Autodesk Inventor part; units mm, degrees
ref_plane "YZ Plane" through (0, 0, 0) normal (1, 0, 0) x (0, 1, 0)
ref_plane "XZ Plane" through (0, 0, 0) normal (0, 1, 0) x (-1, 0, 0)
ref_plane "XY Plane" through (0, 0, 0) normal (0, 0, 1) x (1, 0, 0)
sketch "Skizze1" plane through (0, 0, 0) normal (0, 1, 0) x (-1, 0, 0)
  line L0 (0, 6.5) -> (5.6292, 3.25)
  line L1 (5.6292, 3.25) -> (5.6292, -3.25)
  line L2 (5.6292, -3.25) -> (0, -6.5)
  line L3 (0, -6.5) -> (-5.6292, -3.25)
  line L4 (-5.6292, -3.25) -> (-5.6292, 3.25)
  line L5 (-5.6292, 3.25) -> (0, 6.5)
  circle A0 centre (0, 0) radius 5
  dimension "d0" = 10
  dimension "d1" = 13
extrude "Extrusion1" add sketch "Skizze1" along normal mid plane 4
sketch "Skizze2" plane through (0, 2, 0) normal (0, 1, 0) x (1, 0, 0)
  circle A0 centre (0, 0) radius 5
extrude "Extrusion2" add sketch "Skizze2" along normal blind 12
sketch "Skizze3" plane through (0, 2, 0) normal (0, -1, 0) x (1, 0, 0)
  circle A0 centre (0, 0) radius 5
extrude "Extrusion3" add sketch "Skizze3" along normal blind 13
thread "Gewinde1"
thread "Gewinde2"
sketch "Skizze4" plane through (0, 14, 0) normal (0, 1, 0) x (1, 0, 0)
  circle A0 centre (0, 0) radius 3.5
  dimension "d12" = 7
extrude "Extrusion4" cut sketch "Skizze4" against normal up to surface (25 mm away)
properties part number "1154"
The model under review builds one solid part; all positions refer to its coordinate system, in mm. A direction names the side the tool comes from. Round coordinates to 2 decimals unless told otherwise and drop trailing zeros. Order: outer loops, then holes, each group sorted by start corner. A loop starts at its lowest first (then second) coordinate and runs counter-clockwise, first axis right, second up. Notation, with made-up numbers: (-25, -19.5) -> (-5, -19.5) arc R5 cw to (-5, -15.5) -> close; hole circle Ø4 at (-19, 48.25). An arc over 180 degrees is marked (long way). Return JSON: item names as keys, results as strings.
1. Take a section at D-D (x = 4.5). Write out the cut boundary in (y, z), then the cut area to 3 significant figures.
Answer block:
{"outline": "(-11, -2.18) -> (-2, -2.18) -> (-2, -3.9) -> (2, -3.9) -> (2, -2.18) -> (14, -2.18) -> (14, 2.18) -> (2, 2.18) -> (2, 3.9) -> (-2, 3.9) -> (-2, 2.18) -> (-11, 2.18) -> close", "area": "123 mm²"}
2. For faces 1 (the face through (5, -2, 2)), 2 (the face through (5, 2, 2)), 3 (the face through (-5.629, 0, 0)), list the 3-axis set-ups (+Z, -Z, +X, -X, +Y, -Y) from which the entire face can be reached by the end or side of a thin tool; tool diameter is ignored.
Answer block:
{"face 1": "-Y", "face 2": "+Y", "face 3": "+Z, -Z, -X, +Y, -Y"}
3. For L1, parallel to Z at x = 0, y = -3; L2, parallel to X at y = -7, z = -2.5, list the stretches that pass through material, from the lowest coordinate up. Write a range as [from, to].
Answer block:
{"L1": "z = [-5, -3.5], [3.5, 5]", "L2": "x = [-4.33, -2.45], [2.45, 4.33]"}
4. Take a section at A-A (z = 0). Write out the cut boundary in (x, y).
Answer block:
{"outline": "(-5.63, -2) -> (-5, -2) -> (-5, -11) -> (-3.5, -11) -> (-3.5, 14) -> (-5, 14) -> (-5, 2) -> (-5.63, 2) -> close; (3.5, -11) -> (5, -11) -> (5, -2) -> (5.63, -2) -> (5.63, 2) -> (5, 2) -> (5, 14) -> (3.5, 14) -> close"}
5. Insertion check: P1, Ø5, axis at x = 4, y = 9, coming from the +Z side; P2, Ø6, axis at y = -7.5, z = 2.5, coming from the -X side; P3, Ø6.5, axis at x = 0, z = 0, coming from the -Y side; P4, Ø1.5, axis at y = 6, z = -1, coming from the +X side. Each pin has a flat end and moves straight along its axis. Give the tip position at first contact, or say it passes through.
Answer block:
{"P1": "stops at z = 4.77", "P2": "stops at x = -5", "P3": "passes through", "P4": "stops at x = 4.99"}
6. Take a section at C-C (x = 2). Write out the cut boundary in (y, z).
Answer block:
{"outline": "(-11, -4.58) -> (-2, -4.58) -> (-2, -5.35) -> (2, -5.35) -> (2, -4.58) -> (14, -4.58) -> (14, -2.87) -> (-11, -2.87) -> close; (-11, 2.87) -> (14, 2.87) -> (14, 4.58) -> (2, 4.58) -> (2, 5.35) -> (-2, 5.35) -> (-2, 4.58) -> (-11, 4.58) -> close"}
7. Take a section at B-B (y = 1.75). Write out the cut boundary in (x, z).
Answer block:
{"outline": "(-5.63, -3.25) -> (0, -6.5) -> (5.63, -3.25) -> (5.63, 3.25) -> (0, 6.5) -> (-5.63, 3.25) -> close; hole circle Ø7 at (0, 0)"}
